from build123d import *

# Parameters (mm, degrees)
SKETCH2_R           = 1.375
BOSS_EXTRUDE1_DEPTH = 3.125
SKETCH3_R           = 11
BOSS_EXTRUDE2_DEPTH = 4
FILLET1_SIZE        = 3.125
SKETCH4_W           = 31.47
SKETCH4_H           = 41.76
SKETCH4_W_2         = 25.12
SKETCH4_H_2         = 35.41
BOSS_EXTRUDE3_DEPTH = 49.135
CHAMFER1_SIZE       = 2.38
CHAMFER1_SIZE_2     = 2.597314233
BOSS_EXTRUDE4_DEPTH = 3.175
SKETCH6_W           = 40
SKETCH6_H           = 31.47
CUT_EXTRUDE1_DEPTH  = 3.175
CHAMFER2_SIZE       = 3.175
FILLET3_R           = 5
FILLET4_R           = 5
FILLET5_R           = 1.5


# Some blends are built 0.0001 mm under size
with BuildPart() as part:
    # Sketch2 → Boss-Extrude1 (new body)
    with BuildSketch(Plane(origin=(0, 0, 0), x_dir=(0, 0, -1), z_dir=(1, 0, 0))):
        Polygon((0, 15.615), (-8.5, 15.615), (-15.735, 9), (-15.735, 0), (-15.735, -9), (-8.5, -15.615), (0, -15.615), (8.5, -15.615), (15.735, -9), (15.735, 0), (15.735, 9), (8.5, 15.615), align=None)
        with Locations((0, 7)):
            Circle(SKETCH2_R, mode=Mode.SUBTRACT)
        with Locations((-7, 0)):
            Circle(SKETCH2_R, mode=Mode.SUBTRACT)
        with Locations((7, 0)):
            Circle(SKETCH2_R, mode=Mode.SUBTRACT)
        with Locations((0, -7)):
            Circle(SKETCH2_R, mode=Mode.SUBTRACT)
    extrude(amount=BOSS_EXTRUDE1_DEPTH)

    # Sketch3 → Boss-Extrude2 (add)
    with BuildSketch(Plane.ZY.offset(-3.125)):
        Polygon((-15.735, -9), (-15.735, -26.145), (15.735, -26.145), (15.735, -9), (15.735, 9), (15.735, 15.615), (8.5, 15.615), (-8.5, 15.615), (-15.735, 15.615), (-15.735, 9), align=None)
        Circle(SKETCH3_R, mode=Mode.SUBTRACT)
    extrude(amount=-BOSS_EXTRUDE2_DEPTH)

    # Fillet1
    fillet1_edges = [part.edges().sort_by_distance(p)[0] for p in [
        (3.125, 12.3075, 12.1175),
        (3.125, 12.3075, -12.1175),
        (3.125, -12.3075, -12.1175),
        (3.125, -15.615, 0),
        (3.125, -12.3075, 12.1175),
    ]]
    chamfer(fillet1_edges, length=FILLET1_SIZE - 0.0001)  # a hair under: the kernel refuses the full size

    # Sketch4 → Boss-Extrude3 (add)
    with BuildSketch(Plane(origin=(7.125, 0, 0), x_dir=(0, 0, -1), z_dir=(1, 0, 0))):
        with Locations((0, -5.265)):
            Rectangle(SKETCH4_W, SKETCH4_H)
        with Locations((0, -5.265)):
            Rectangle(SKETCH4_W_2, SKETCH4_H_2, mode=Mode.SUBTRACT)
    extrude(amount=BOSS_EXTRUDE3_DEPTH)

    # Chamfer1
    # the kernel refuses this chamfer: 2.597314233, 2.38 mm, written as the material it takes off along each edge
    with BuildSketch(Plane(origin=(-3.562082301, 15.615, 15.735), x_dir=(0, 0.031246667353746232, -0.9995117036729906), z_dir=(1, 0, 0))) as chamfer1_piece_1:
        Polygon((CHAMFER1_SIZE * 0.999511703673, -CHAMFER1_SIZE * 0.0312466673537), (-CHAMFER1_SIZE_2 * 0.0312466673483, -CHAMFER1_SIZE_2 * 0.999511703498), (0, 0), align=None)
    extrude(amount=66.509164603, mode=Mode.SUBTRACT)
    with BuildSketch(Plane(origin=(62.947082301, 15.615, -15.735), x_dir=(0, 0.02624044362699192, 0.999655660274206), z_dir=(-1, 0, 0))) as chamfer1_piece_2:
        Polygon((CHAMFER1_SIZE_2 * 0.999655660099, -CHAMFER1_SIZE_2 * 0.0262404436224), (-CHAMFER1_SIZE * 0.026240443627, -CHAMFER1_SIZE * 0.999655660274), (0, 0), align=None)
    extrude(amount=66.509164603, mode=Mode.SUBTRACT)

    # Sketch5 → Boss-Extrude4 (add)
    with BuildSketch(Plane(origin=(56.26, 0, 0), x_dir=(0, 0, -1), z_dir=(1, 0, 0))):
        Polygon((13.137685767, 15.615), (-13.355, 15.615), (-15.735, 13.017685767), (-15.735, -26.145), (15.735, -26.145), (15.735, 13.235), align=None)
    extrude(amount=BOSS_EXTRUDE4_DEPTH)

    # Sketch6 → Cut-Extrude1 (cut)
    with BuildSketch(Plane.XZ.offset(26.145)):
        with Locations((39.435, 0)):
            Rectangle(SKETCH6_W, SKETCH6_H)
    extrude(amount=-CUT_EXTRUDE1_DEPTH, mode=Mode.SUBTRACT)

    # Chamfer2
    chamfer2_edges = [part.edges().sort_by_distance(p)[0] for p in [
        (19.435, -26.145, 0),
    ]]
    chamfer(chamfer2_edges, length=CHAMFER2_SIZE - 0.0001)  # a hair under: the kernel refuses the full size

    # Fillet3
    fillet3_edges = [part.edges().sort_by_distance(p)[0] for p in [
        (59.435, 15.615, 0.108657116),
    ]]
    fillet(fillet3_edges, radius=FILLET3_R)

    # Fillet4
    # the kernel refuses this fillet: 5 mm, written as the material it takes off along each edge
    with BuildSketch(Plane(origin=(59.435, -22.97, -28.235), x_dir=(0, 1, 0), z_dir=(0, 0, 1))) as fillet4_piece_1:
        with BuildLine():
            CenterArc((FILLET4_R, FILLET4_R), FILLET4_R, 180, 90)
            Line((0, FILLET4_R), (0, 0))
            Line((0, 0), (FILLET4_R, 0))
        make_face()
    extrude(amount=56.47, mode=Mode.SUBTRACT)

    # Fillet5
    fillet5_edges = [part.edges().sort_by_distance(p)[0] for p in [
        (0, 15.615, 0),
    ]]
    fillet(fillet5_edges, radius=FILLET5_R)


solid = part.part
Work out the finished part from the listing and answer in its coordinate system (mm). A direction names the side the tool comes from. Round coordinates to 2 decimals unless told otherwise and drop trailing zeros. Write each loop counter-clockwise with the first axis right and the second up, starting at its lowest first coordinate (ties: lowest second). Pieces come first, ordered by that corner, then holes. Notation, with made-up numbers: (85.5, -2.5) - (132.5, -2.5) arc R16 cw to (132.5, 6.5) - close; hole circle Ø2 at (7, -26). An arc over 180 degrees is marked (long way). Answer in a Markdown table with one row per item. Add a question column.
1. Given pin 1 (2 mm diameter, centred on y = 0, z = -7, fed in from -X); pin 2 (2.5 mm diameter, centred on x = 44.5, z = -13.5, fed in from -Y); pin 3 (1.5 mm diameter, centred on x = 51, z = -9, fed in from -Y), each flat-ended and moving along its own axis, determine where each tip first touches the part or whether it passes through.
2. A cutting plane is placed at B-B, the plane y = 0. Determine the outline of the cut face in (x, z) (3 decimals).
3. A cutting plane is placed at A-A, the plane z = 0. Count the separate pieces of the cut face and the enclosed holes in it, and give its area (3 significant figures).
4. For faces 4 (the flat face through (56.26, -5, 0)), 5 (the cylindrical face through (1.541, 8.363, 0.179)), 6 (the cylindrical face through (0.428, 15.164, 0.15)), 7 (the flat face through (37, -22.97, -14)), 8 (the flat face through (7.125, -13, 0)), determine the directions among +Z, -Z, +X, -X, +Y, -Y from which every point of the face is accessible in a straight line to the end or side of a thin tool.
5. Find the intervals of material crossed by line 1 along X through (y, z) = (6.5, 10.5) (3 decimals); line 2 along Z through (x, y) = (16.5, -2.5) (3 decimals); line 3 along X through (y, z) = (-2.5, -6) (3 decimals), in increasing order. Write a range as from..to.
6. A cutting plane is placed at D-D, the plane x = 21. Determine the outline of the cut face in (y, z) (3 decimals), and give its area (3 significant figures).
7. The mould has two halves that part along Z. Classify faces 1 (the flat face through (28, 15.615, 0)), 2 (the flat face through (1.19, 12.86, 13.28)), 3 (the cylindrical face through (1.541, -5.637, 0.179)): +Z half, -Z half, draft (parallel to the pull), parting line (faces both ways), or undercut.
8. A cutting plane is placed at C-C, the plane x = 14.5. Determine the outline of the cut face in (y, z) (3 decimals).
Worked out:
| question | item | result |
|---|---|---|
| 1 | pin 1 | x = 56.26 |
| 1 | pin 2 | y = -22.97 |
| 1 | pin 3 | y = 12.44 |
| 2 | outline | (0, -15.735) - (59.435, -15.735) - (59.435, 15.735) - (0, 15.735) - (0, 8.375) - (3.125, 8.375) - (3.125, 11) - (7.125, 11) - (7.125, 12.56) - (56.26, 12.56) - (56.26, -12.56) - (7.125, -12.56) - (7.125, -11) - (3.125, -11) - (3.125, -8.375) - (0, -8.375) - close; (0, -5.625) - (3.125, -5.625) - (3.125, 5.625) - (0, 5.625) - close |
| 3 | separate pieces | 3 |
| 3 | enclosed holes | 0 |
| 3 | area | 466 mm^2 |
| 4 | face 4 | -Y |
| 4 | face 5 | -X |
| 4 | face 6 | +Z, -Z, -X, +Y |
| 4 | face 7 | +Z, -Z, +X, -Y |
| 4 | face 8 | none |
| 5 | line 1 | 0..7.125, 56.26..59.435 |
| 5 | line 2 | -15.735..-12.56, 12.56..15.735 |
| 5 | line 3 | 0..3.125, 56.26..59.435 |
| 6 | outline | (-22.97, -15.735) - (13.235, -15.735) - (15.615, -13.138) - (15.615, 13.355) - (13.018, 15.735) - (-22.97, 15.735) - (-22.97, 12.56) - (12.44, 12.56) - (12.44, -12.56) - (-22.97, -12.56) - close |
| 6 | area | 319 mm^2 |
| 7 | face 1 | draft |
| 7 | face 2 | +Z half |
| 7 | face 3 | undercut |
| 8 | outline | (-26.145, -15.735) - (13.235, -15.735) - (15.615, -13.138) - (15.615, 13.355) - (13.018, 15.735) - (-26.145, 15.735) - close; hole (-22.97, -12.56) - (12.44, -12.56) - (12.44, 12.56) - (-22.97, 12.56) - close |
